Could you check a few things on this drawing? It's one solid part, dimensions in mm from its lowest x, y, z. A direction names the side the tool comes from. Round coordinates to 2 decimals unless told otherwise and drop trailing zeros. Loops run counter-clockwise (first coordinate to the right, second up) from the corner with the lowest first, then second, coordinate; pieces in that order, holes last. Notation, with made-up numbers: (17, 34.5) -> (29, 34.5) arc R23 ccw to (29, 72.5) -> close; hole circle Ø3 at (82.5, 29.25). An arc over 180 degrees is marked (long way). Put each result on its own line as item: value. Start each with the question number.
1. Imagine slicing it at B-B, the plane z = 20.5. Count the separate pieces of the cut face and the enclosed holes in it, and give its area (3 significant figures).
2. I need wall thicknesses on line 1 (X direction, y = 1.3, z = 20.5); line 2 (Z direction, x = 3.35, y = 0.8); line 3 (Z direction, x = 16.5, y = 4.75). Which ranges of each line are inside material? Lowest first, please. Write a range as [from, to].
3. Imagine slicing it at C-C, the plane x = 29.5. Please give me the cut outline in (y, z).
4. Imagine slicing it at A-A, the plane x = 21.85. Please give me the cut outline in (y, z), and give its area (3 significant figures).
5. I'm going to push flat-ended pins straight in: P1, Ø3, axis at x = 22, z = 22.5, coming from the +Y side; P2, Ø5, axis at y = 9, z = 19.5, coming from the +X side; P3, Ø7, axis at y = 5, z = 30, coming from the +X side; P4, Ø2.5, axis at x = 56.85, z = 20.5, coming from the -Y side. Where does each tip first touch, or does it pass through?
6. If we mould it in two halves opening along Z, with no side actions, what happens to the marked faces 1, 2 and 3? For each: pulls with the +Z half, pulls with the -Z half, needs draft (parallel to the pull), parting line crosses it, or undercut.
7. Which directions (+Z, -Z, +X, -X, +Y, -Y) give clear straight access to the entire face, cutting with the end or side of a thin tool? Please do the marked faces 4, 5, 6, 7 and 8.
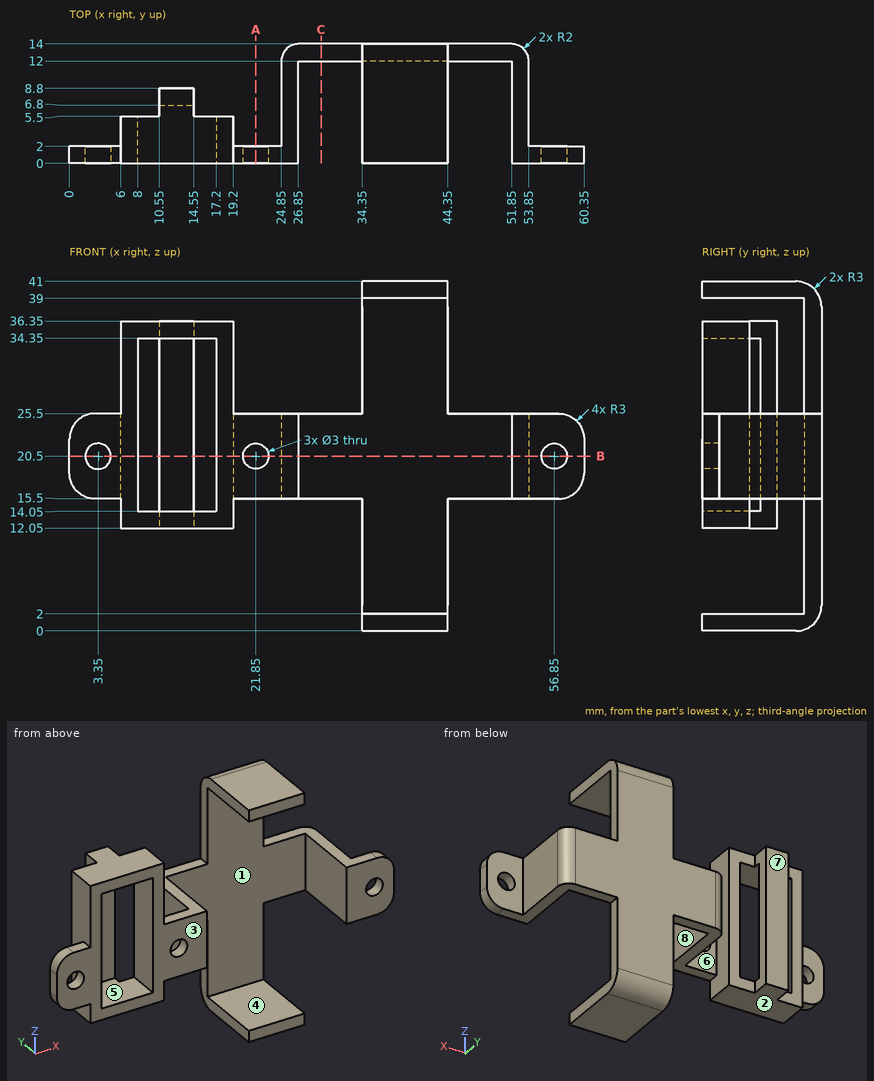
Entries:
1. separate pieces: 6
1. enclosed holes: 0
1. area: 153 mm^2
2. line 1: [0, 1.85], [4.85, 8], [17.2, 20.35], [23.35, 26.85], [51.85, 55.35], [58.35, 60.35]
2. line 2: [15.5, 19], [22, 25.5]
2. line 3: [12.05, 14.05], [34.35, 36.35]
3. outline: (12, 15.5) -> (14, 15.5) -> (14, 25.5) -> (12, 25.5) -> close
4. outline: (0, 15.5) -> (2, 15.5) -> (2, 19) -> (0, 19) -> close; (0, 22) -> (2, 22) -> (2, 25.5) -> (0, 25.5) -> close
4. area: 14.0 mm^2
5. P1: y = 2
5. P2: x = 53.85
5. P3: x = 19.2
5. P4: through
6. face 1: undercut
6. face 2: pulls with the -Z half
6. face 3: needs draft
7. face 4: +X, -X, -Y
7. face 5: -Y
7. face 6: +Z, -Z, +Y
7. face 7: +Z, -Z, -X, +Y
7. face 8: +Z, -Z, -Y
